from build123d import *

# Parameters (mm, degrees)
SKETCH1_W                                            = 16.1
SKETCH1_H                                            = 14.1
BOSS_EXTRUDE1_DEPTH                                  = 10.6
SKETCH3_W                                            = 12.1
SKETCH3_H                                            = 10.1
CUT_EXTRUDE1_DEPTH                                   = 8.6
CSK_FOR_M1_6_COUNTERSUNK_FLAT_HEAD_SCREW_D           = 2
CSK_FOR_M1_6_COUNTERSUNK_FLAT_HEAD_SCREW_DEPTH       = 2
CSK_FOR_M1_6_COUNTERSUNK_FLAT_HEAD_SCREW_CSINK_D     = 4
CSK_FOR_M1_6_COUNTERSUNK_FLAT_HEAD_SCREW_CSINK_ANGLE = 90
SKETCH8_R                                            = 2.25
CUT_EXTRUDE2_DEPTH                                   = 3
FILLET2_R                                            = 0.2
SKETCH9_W                                            = 15
SKETCH9_H                                            = 14.1
BOSS_EXTRUDE2_DEPTH                                  = 2


with BuildPart() as part:
    # Sketch1 → Boss-Extrude1 (new body)
    with BuildSketch(Plane(origin=(0, 0, 0), x_dir=(1, 0, 0), z_dir=(0, 1, 0))):
        Rectangle(SKETCH1_W, SKETCH1_H)
    extrude(amount=BOSS_EXTRUDE1_DEPTH)

    # Sketch3 → Cut-Extrude1 (cut)
    with BuildSketch(Plane(origin=(0, 10.6, 0), x_dir=(1, 0, 0), z_dir=(0, 1, 0))):
        Rectangle(SKETCH3_W, SKETCH3_H)
    extrude(amount=-CUT_EXTRUDE1_DEPTH, mode=Mode.SUBTRACT)

    # CSK for M1.6 Countersunk Flat Head Screw1
    with Locations(Plane(origin=(0, 0, 0), x_dir=(-1, 0, 0), z_dir=(0, -1, 0))):
        with Locations((4.5, 0), (-4.5, 0)):
            CounterSinkHole(CSK_FOR_M1_6_COUNTERSUNK_FLAT_HEAD_SCREW_D / 2, CSK_FOR_M1_6_COUNTERSUNK_FLAT_HEAD_SCREW_CSINK_D / 2, depth=CSK_FOR_M1_6_COUNTERSUNK_FLAT_HEAD_SCREW_DEPTH, counter_sink_angle=CSK_FOR_M1_6_COUNTERSUNK_FLAT_HEAD_SCREW_CSINK_ANGLE)

    # Sketch8 → Cut-Extrude2 (cut, through all)
    with BuildSketch(Plane(origin=(0, 2, 0), x_dir=(1, 0, 0), z_dir=(0, 1, 0))):
        Circle(SKETCH8_R)
    extrude(amount=-CUT_EXTRUDE2_DEPTH, mode=Mode.SUBTRACT)

    # Fillet2
    fillet2_edges = [part.edges().sort_by_distance(p)[0] for p in [
        (-6.05, 6.3, 5.05),
        (-6.05, 6.3, -5.05),
        (6.05, 6.3, -5.05),
        (6.05, 6.3, 5.05),
    ]]
    fillet(fillet2_edges, radius=FILLET2_R)

    # Sketch9 → Boss-Extrude2 (add)
    with BuildSketch(Plane(origin=(0, 0, 0), x_dir=(1, 0, 0), z_dir=(0, 1, 0))):
        with Locations((-15.55, 0)):
            Rectangle(SKETCH9_W, SKETCH9_H)
    boss_extrude2 = extrude(amount=BOSS_EXTRUDE2_DEPTH)

    # Sketch11 → CSK for M4 Countersunk Flat Head Screw1 (revolve, cut)
    with BuildSketch(Plane(origin=(-16, 2, 0), x_dir=(0, 0, 1), z_dir=(1, 0, 0))):
        Polygon((0, 0), (0, 2.001), (2.4, 2.001), (2.4, 2.3), (4.7, 0), align=None)
    csk_for_m4_countersunk_flat_head_screw1 = revolve(axis=Axis((-16, 8.35, 0), (0, -1, 0)), mode=Mode.SUBTRACT)

    # Mirror1: Boss-Extrude2, CSK for M4 Countersunk Flat Head Screw1 across plane
    add(boss_extrude2.mirror(Plane(origin=(0, 0, 0), x_dir=(0, 0, 1), z_dir=(1, 0, 0))))
    add(csk_for_m4_countersunk_flat_head_screw1.mirror(Plane(origin=(0, 0, 0), x_dir=(0, 0, 1), z_dir=(1, 0, 0))), mode=Mode.SUBTRACT)


solid = part.part
Build history of the part. All positions in model axes, mm. A direction names the side the tool comes from. Round coordinates to 2 decimals unless told otherwise and drop trailing zeros. Loops run counter-clockwise (first coordinate to the right, second up) from the corner with the lowest first, then second, coordinate; pieces in that order, holes last. Notation, with made-up numbers: (-29, 43) -> (-9, 43) arc R19 cw to (-9, 49) -> close; hole circle Ø6 at (73, 47). An arc over 180 degrees is marked (long way). Answer in a Markdown table with one row per item.
Item 1: Drill centre lines: L1, parallel to X at y = 8, z = 4.5; L2, parallel to Z at x = -4.5, y = 1.35; L3, parallel to X at y = 1.5, z = -0.75. Where is each one in solid material? Low to high. Write a range as [from, to].
Answers below:
| item | result |
|---|---|
| L1 | x = [-8.05, -6.05], [6.05, 8.05] |
| L2 | z = [-7.05, -1], [1, 7.05] |
| L3 | x = [-23.05, -20.13], [-11.87, -5.16], [-3.84, -2.12], [2.12, 3.84], [5.16, 11.87], [20.13, 23.05] |
Item 2: Saw through at A-A (x = -16). Write the cut outline in (y, z).
Answers below:
| item | result |
|---|---|
| outline | (0, -7.05) -> (2, -7.05) -> (2, -4.7) -> (0, -2.7) -> close; (0, 2.7) -> (2, 4.7) -> (2, 7.05) -> (0, 7.05) -> close |
Item 3: Saw through at B-B (y = 3.5). Write the cut outline in (x, z).
Answers below:
| item | result |
|---|---|
| outline | (-8.05, -7.05) -> (8.05, -7.05) -> (8.05, 7.05) -> (-8.05, 7.05) -> close; hole (-6.05, -4.85) arc R0.2 ccw to (-5.85, -5.05) -> (5.85, -5.05) arc R0.2 ccw to (6.05, -4.85) -> (6.05, 4.85) arc R0.2 ccw to (5.85, 5.05) -> (-5.85, 5.05) arc R0.2 ccw to (-6.05, 4.85) -> close |
Item 4: Which spindle directions (+Z, -Z, +X, -X, +Y, -Y) get a long thin tool onto all of the face, cutting with end or side? Do faces 1 (the flat face through (0, 6, -5.05)), 2 (the flat face through (8.05, 6, 0)), 3 (the flat face through (-12, 2, -3)). Say none if no direction does.
Answers below:
| item | result |
|---|---|
| face 1 | +Y |
| face 2 | +Z, -Z, +X, +Y |
| face 3 | +Z, -Z, -X, +Y |
Item 5: Pin check, flat tips, straight feed: pin 1 (2.5 mm diameter, centred on x = -4.5, z = 0, fed in from -Y); pin 2 (6 mm diameter, centred on y = 4, z = -5, fed in from -X); pin 3 (3.5 mm diameter, centred on x = 0, z = 0, fed in from -Y); pin 4 (6 mm diameter, centred on x = 18, z = -2.5, fed in from +Y). Stop position of each tip, or through.
Answers below:
| item | result |
|---|---|
| pin 1 | stops at y = 0.75 |
| pin 2 | stops at x = -23.05 |
| pin 3 | passes through |
| pin 4 | stops at y = 2 |
Item 6: Mould opens along Z. For faces 4 (the flat face through (0, 4, 7.05)), 5 (the flat face through (-8.05, 6, 0)), 6 (the flat face through (-1.4, 2, -2.3)) say: +Z half, -Z half, draft (parallel to the pull), parting line (faces both ways), or undercut.
Answers below:
| item | result |
|---|---|
| face 4 | +Z half |
| face 5 | draft |
| face 6 | undercut |
Item 7: Saw through at D-D (x = 4.5). Write the cut outline in (y, z), and give its area (3 significant figures).
Answers below:
| item | result |
|---|---|
| outline | (0, -7.05) -> (10.6, -7.05) -> (10.6, -5.05) -> (2, -5.05) -> (2, -1) -> (1, -1) -> (0, -2) -> close; (0, 2) -> (1, 1) -> (2, 1) -> (2, 5.05) -> (10.6, 5.05) -> (10.6, 7.05) -> (0, 7.05) -> close |
| area | 57.6 mm² |
Item 8: Saw through at C-C (z = 6). Write the cut outline in (x, y), and give its area (3 significant figures).
Answers below:
| item | result |
|---|---|
| outline | (-23.05, 0) -> (23.05, 0) -> (23.05, 2) -> (8.05, 2) -> (8.05, 10.6) -> (-8.05, 10.6) -> (-8.05, 2) -> (-23.05, 2) -> close |
| area | 231 mm² |
